Build history of the part. All positions in model axes, mm. Face numbers are marked on the shaded views. A direction names the side the tool comes from. Round coordinates to 2 decimals unless told otherwise and drop trailing zeros. Order: outer loops, then holes, each group sorted by start corner. A loop starts at its lowest first (then second) coordinate and runs counter-clockwise, first axis right, second up. Notation, with made-up numbers: (69, -12.75) -> (90, -12.75) arc R16 cw to (90, 6.25) -> close; hole circle Ø9 at (58, 64). An arc over 180 degrees is marked (long way). Answer as a JSON object with one key per item and string values.
from build123d import *

# Parameters (mm, degrees)
SKETCH1_W           = 101.6
SKETCH1_H           = 101.6
BOSS_EXTRUDE1_DEPTH = 304.8
SKETCH2_W           = 50.8
SKETCH2_H           = 101.6
SKETCH2_W_2         = 101.6
SKETCH2_H_2         = 50.8
CUT_EXTRUDE3_DEPTH  = 101.6


with BuildPart() as part:
    # Sketch1 → Boss-Extrude1 (new body)
    with BuildSketch(Plane(origin=(0, 0, 0), x_dir=(1, 0, 0), z_dir=(0, 1, 0))):
        Rectangle(SKETCH1_W, SKETCH1_H)
    extrude(amount=BOSS_EXTRUDE1_DEPTH)

    # Sketch2 → Cut-Extrude3 (cut)
    with BuildSketch(Plane(origin=(0, 304.8, 0), x_dir=(1, 0, 0), z_dir=(0, 1, 0))):
        Rectangle(SKETCH2_W, SKETCH2_H)
        Rectangle(SKETCH2_W_2, SKETCH2_H_2)
    extrude(amount=-CUT_EXTRUDE3_DEPTH, mode=Mode.SUBTRACT)


solid = part.part
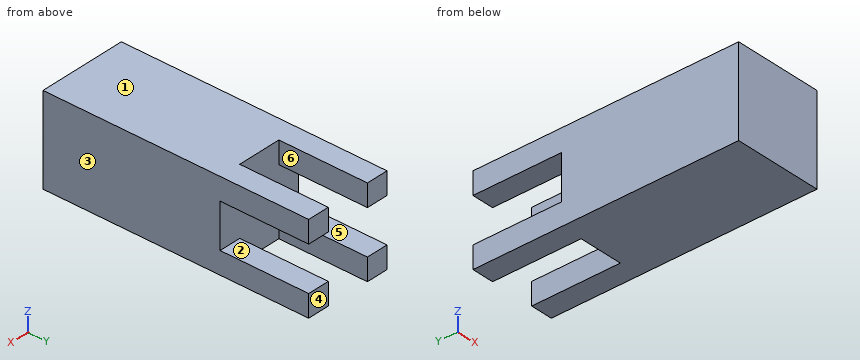
1) Cut at B-B, the plane z = 34.5. Give the cut face in (x, y), plus the area to 3 significant figures.
Checked values:
{"outline": "(-50.8, 0) -> (50.8, 0) -> (50.8, 304.8) -> (25.4, 304.8) -> (25.4, 203.2) -> (-25.4, 203.2) -> (-25.4, 304.8) -> (-50.8, 304.8) -> close", "area": "25,800 mm²"}
2) Cut at C-C, the plane x = 29. Give the cut face in (y, z).
Checked values:
{"outline": "(0, -50.8) -> (304.8, -50.8) -> (304.8, -25.4) -> (203.2, -25.4) -> (203.2, 25.4) -> (304.8, 25.4) -> (304.8, 50.8) -> (0, 50.8) -> close"}
3) Which spindle directions (+Z, -Z, +X, -X, +Y, -Y) get a long thin tool onto all of the face, cutting with end or side? Do the marked faces 4, 5 and 6. Say none if no direction does.
Checked values:
{"face 4": "+Z, -Z, +X, -X, +Y", "face 5": "+X, -X, +Y", "face 6": "+Z, -Z, +Y"}
4) Pull direction Z, two halves, no side cores. Call the marked faces 1, 2 and 3: pulls with the +Z half, pulls with the -Z half, needs draft (parallel to the pull), parting line crosses it, or undercut.
Checked values:
{"face 1": "pulls with the +Z half", "face 2": "undercut", "face 3": "needs draft"}
5) Cut at D-D, the plane z = 15. Give the cut face in (x, y), plus the area to 3 significant figures.
Checked values:
{"outline": "(-50.8, 0) -> (50.8, 0) -> (50.8, 203.2) -> (-50.8, 203.2) -> close", "area": "20,600 mm²"}
6) Probe L1, parallel to Z at x = 31.5, y = 207; L2, parallel to Y at x = -8.5, z = 24.5. List the from-to ranges inside material, lowest first. Write a range as from..to.
Checked values:
{"L1": "z = -50.8..-25.4, 25.4..50.8", "L2": "y = 0..203.2"}
7) Flat gauge pins, fed straight in: pin 1 Ø1 at (x, y) = (23, 230) entering from -Z; pin 2 Ø3 at (x, z) = (20, -20.5) entering from +Y. Where does each tip first touch, or does it go through?
Checked values:
{"pin 1": "passes through", "pin 2": "stops at y = 203.2"}
8) Cut at A-A, the plane y = 216.5. Give the cut face in (x, z).
Checked values:
{"outline": "(-50.8, -50.8) -> (-25.4, -50.8) -> (-25.4, -25.4) -> (-50.8, -25.4) -> close; (-50.8, 25.4) -> (-25.4, 25.4) -> (-25.4, 50.8) -> (-50.8, 50.8) -> close; (25.4, -50.8) -> (50.8, -50.8) -> (50.8, -25.4) -> (25.4, -25.4) -> close; (25.4, 25.4) -> (50.8, 25.4) -> (50.8, 50.8) -> (25.4, 50.8) -> close"}
